```python
from build123d import *

# Parameters (mm, degrees)
SKETCH1_R           = 32.5
BOSS_EXTRUDE1_DEPTH = 35
SKETCH2_W           = 10.1
SKETCH2_H           = 15.1
CUT_EXTRUDE1_DEPTH  = 5.1
SKETCH3_R           = 7
CUT_EXTRUDE2_DEPTH  = 58.771100041
SKETCH4_W           = 17
SKETCH4_H           = 7
CUT_EXTRUDE3_DEPTH  = 15
FILLET1_R           = 2.5


with BuildPart() as part:
    # Sketch1 → Boss-Extrude1 (new body)
    with BuildSketch(Plane(origin=(0, 0, 0), x_dir=(1, 0, 0), z_dir=(0, 1, 0))):
        with Locations(Location((0, 0, 0), (0, 0, 270))):
            Circle(SKETCH1_R)
    extrude(amount=BOSS_EXTRUDE1_DEPTH)

    # Sketch2 → Cut-Extrude1 (cut)
    with BuildSketch(Plane(origin=(0, 35, 0), x_dir=(1, 0, 0), z_dir=(0, 1, 0))):
        with Locations((0, 22.45)):
            Rectangle(SKETCH2_W, SKETCH2_H)
        with Locations((0, -22.45)):
            Rectangle(SKETCH2_W, SKETCH2_H)
    extrude(amount=-CUT_EXTRUDE1_DEPTH, mode=Mode.SUBTRACT)

    # Sketch3 → Cut-Extrude2 (cut, through all)
    with BuildSketch(Plane(origin=(0, 35, 0), x_dir=(1, 0, 0), z_dir=(0, 1, 0))):
        with Locations(Location((0, 0, 0), (0, 0, 270))):
            Circle(SKETCH3_R)
    extrude(amount=-CUT_EXTRUDE2_DEPTH, mode=Mode.SUBTRACT)

    # Sketch4 → Cut-Extrude3 (cut)
    with BuildSketch(Plane(origin=(0, 35, 0), x_dir=(1, 0, 0), z_dir=(0, 1, 0))):
        with Locations((19.746175473, 0)):
            Rectangle(SKETCH4_W, SKETCH4_H)
        with Locations((-19.746175473, 0)):
            Rectangle(SKETCH4_W, SKETCH4_H)
    extrude(amount=-CUT_EXTRUDE3_DEPTH, mode=Mode.SUBTRACT)

    # Fillet1
    fillet1_edges = [part.edges().sort_by_distance(p)[0] for p in [
        (28.246175473, 35, 0),
        (19.746175473, 35, -3.5),
        (11.246175473, 35, 0),
        (19.746175473, 35, 3.5),
        (-19.746175473, 35, 3.5),
        (-11.246175473, 35, 0),
        (-19.746175473, 35, -3.5),
        (-28.246175473, 35, 0),
    ]]
    fillet(fillet1_edges, radius=FILLET1_R)


solid = part.part
```
The model under review builds one solid part; all positions refer to its coordinate system, in mm. A direction names the side the tool comes from. Round coordinates to 2 decimals unless told otherwise and drop trailing zeros. Write each loop counter-clockwise with the first axis right and the second up, starting at its lowest first coordinate (ties: lowest second). Pieces come first, ordered by that corner, then holes. Notation, with made-up numbers: M 26.25,38 L 74.25,38 A22 ccw 74.25,50 Z; hole C -14.5,46.5 d10. An arc over 180 degrees is marked long. Use CSV: the item, a comma, the result in double quotes. Start each with the question number.
(1) We need section D-D, the plane z = -21.5. State the section outline as (x, y) points, then the cut area to 3 significant figures.
(2) Clearance check with flat-ended pins moving along their axes: P1, Ø11, axis at x = -2, z = -19, coming from the +Y side; P2, Ø1, axis at y = 28.5, z = 17.5, coming from the +X side; P3, Ø3.5, axis at x = 19, z = 1, coming from the +Y side; P4, Ø8, axis at x = -8, y = 27, coming from the -Z side. State where each tip first meets the part, or that it passes through.
(3) Tool access review of faces 1 (the face through (-20, 20, 0)), 2 (the face through (-6.834, 17.745, -1.517)): name each direction out of +Z, -Z, +X, -X, +Y, -Y from which nothing blocks a thin tool from reaching the whole face with its end or side.
(4) The part is to be moulded in two halves that separate along X. For faces 3 (the face through (28.246, 26, 0)), 4 (the face through (8, 0, 0)), say which applies: +X half, -X half, draft (parallel to the pull), parting line (faces both ways), or undercut.
(5) We need section C-C, the plane y = 8.5. State the section outline as (x, z) points.
(6) We need section A-A, the plane z = 0. State the section outline as (x, y) points, then the cut area to 3 significant figures.
(7) We need section B-B, the plane x = 0. State the section outline as (y, z) points.
(8) For line 1 along X through (y, z) = (24, 0); line 2 along X through (y, z) = (17.5, 0); line 3 along X through (y, z) = (26.5, 2), list the stretches that pass through material, from the lowest coordinate up.
Findings:
1,outline,"M -24.37,0 L 24.37,0 L 24.37,35 L 5.05,35 L 5.05,29.9 L -5.05,29.9 L -5.05,35 L -24.37,35 Z"
1,area,"1,650 mm^2"
2,P1,"y = 35"
2,P2,"x = 27.7"
2,P3,"y = 20"
2,P4,"z = -32.25"
3,face 1,"+Y"
3,face 2,"+Y, -Y"
4,face 3,"undercut"
4,face 4,"draft"
5,outline,"C 0,0 d65; hole C 0,0 d14"
6,outline,"M -32.5,0 L -7,0 L -7,35 L -8.75,35 A2.5 ccw -11.25,32.5 L -11.25,20 L -28.25,20 L -28.25,32.5 A2.5 ccw -30.75,35 L -32.5,35 Z; M 7,0 L 32.5,0 L 32.5,35 L 30.75,35 A2.5 ccw 28.25,32.5 L 28.25,20 L 11.25,20 L 11.25,32.5 A2.5 ccw 8.75,35 L 7,35 Z"
6,area,"1,270 mm^2"
7,outline,"M 0,-32.5 L 35,-32.5 L 35,-30 L 29.9,-30 L 29.9,-14.9 L 35,-14.9 L 35,-7 L 0,-7 Z; M 0,7 L 35,7 L 35,14.9 L 29.9,14.9 L 29.9,30 L 35,30 L 35,32.5 L 0,32.5 Z"
8,line 1,"-32.5 to -28.25, -11.25 to -7, 7 to 11.25, 28.25 to 32.5"
8,line 2,"-32.5 to -7, 7 to 32.5"
8,line 3,"-32.44 to -28.25, -11.25 to -6.71, 6.71 to 11.25, 28.25 to 32.44"
